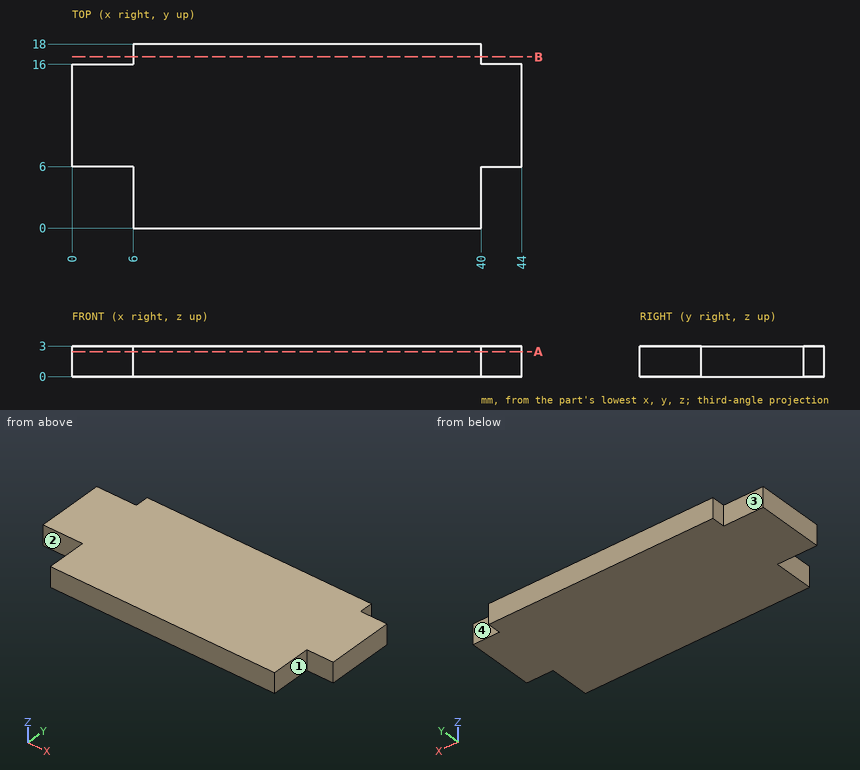
Design review of the part shown in the three views and the two pictorial views. Dimensions are in mm from the part's minimum x, y and z. A direction names the side the tool comes from. Give positions to 0.01 mm unless a question says otherwise; leave off trailing zeros. Write each loop counter-clockwise with the first axis right and the second up, starting at its lowest first coordinate (ties: lowest second). Pieces come first, ordered by that corner, then holes.
(1) Clearance check with a flat-ended pin moving along its axis: pin 1 Ø0.6 at (y, z) = (17.5, 1) entering from -X. State where the tip first meets the part, or that it passes through.
Checked values:
pin 1: stops at x = 6
(2) Tool access review of the marked faces 1, 2, 3 and 4: name each direction out of +Z, -Z, +X, -X, +Y, -Y from which nothing blocks a thin tool from reaching the whole face with its end or side.
Checked values:
face 1: +Z, -Z, +X, -Y
face 2: +Z, -Z, -X, -Y
face 3: +Z, -Z, -X, +Y
face 4: +Z, -Z, +X, +Y
(3) Add section A-A (z = 2.45). Give the boundary of the cut face in (x, y), and give its area (3 significant figures).
Checked values:
outline: (0, 6) - (6, 6) - (6, 0) - (40, 0) - (40, 6) - (44, 6) - (44, 16) - (40, 16) - (40, 18) - (6, 18) - (6, 16) - (0, 16) - close
area: 712 mm2
(4) Wall thickness on line 1 along Y through (x, z) = (42.5, 0.55); line 2 along X through (y, z) = (4.75, 1.15): over which ranges is each line inside the solid? List them lowest first.
Checked values:
line 1: y = 6 to 16
line 2: x = 6 to 40
(5) Add section B-B (y = 16.75). Give the boundary of the cut face in (x, z), and give its area (3 significant figures).
Checked values:
outline: (6, 0) - (40, 0) - (40, 3) - (6, 3) - close
area: 102 mm2
